For this review, use the dimensioned drawing (mm, ordinates from the lowest corner) and the shaded views. Give positions to 0.01 mm unless a question says otherwise; leave off trailing zeros. Loops run counter-clockwise (first coordinate to the right, second up) from the corner with the lowest first, then second, coordinate; pieces in that order, holes last. Notation, with made-up numbers: M -8,72.5 L 17,72.5 A19 ccw 17,90.5 Z; hole C 50,30 d8. An arc over 180 degrees is marked long. Use a Markdown table: item, result. Add a question column.
(1) Draft analysis for pull direction Y (two halves, no side actions). For the marked faces 1, 2, 3 and 4, state which applies: pulls with the +Y half, pulls with the -Y half, needs draft (parallel to the pull), parting line crosses it, or undercut.
(2) Add section C-C, the plane y = 1.75. Give the boundary of the cut face in (x, z).
(3) For probe 1 along Y at (x, z) = (5, 2.2); probe 2 along X at (y, z) = (6.5, 1.75); probe 3 along Z at (x, y) = (28.5, 0.5), list the stretches that pass through material, from the lowest coordinate up.
(4) Add section B-B, the plane z = 2. Give the boundary of the cut face in (x, y), then the cut area to 3 significant figures.
(5) Add section A-A, the plane x = 5. Give the boundary of the cut face in (y, z), then the cut area to 3 significant figures.
(6) Add section D-D, the plane z = 5.25. Give the boundary of the cut face in (x, y), then the cut area to 3 significant figures.
(7) Insertion check: pin 1 Ø5.5 at (x, y) = (23, 5) entering from -Z; pin 2 Ø2 at (y, z) = (2, 6) entering from -X; pin 3 Ø6 at (x, y) = (14.5, 7.5) entering from +Z. Each pin has a flat end and moves straight along its axis. Give the tip position at first contact, or say it passes through.
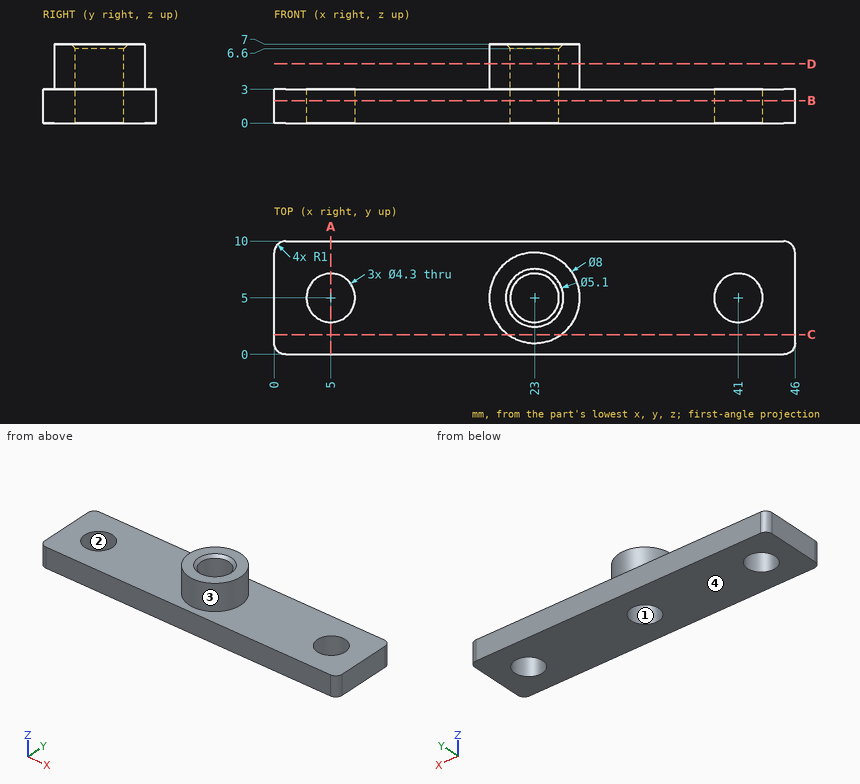
Established:
| question | item | result |
|---|---|---|
| 1 | face 1 | undercut |
| 1 | face 2 | undercut |
| 1 | face 3 | parting line crosses it |
| 1 | face 4 | needs draft |
| 2 | outline | M 0,0 L 46,0 L 46,3 L 25.33,3 L 25.33,7 L 20.67,7 L 20.67,3 L 0,3 Z |
| 3 | probe 1 | 0 to 2.85, 7.15 to 10 |
| 3 | probe 2 | 0 to 3.46, 6.54 to 21.46, 24.54 to 39.46, 42.54 to 46 |
| 3 | probe 3 | 0 to 3 |
| 4 | outline | M 0,1 A1 ccw 1,0 L 45,0 A1 ccw 46,1 L 46,9 A1 ccw 45,10 L 1,10 A1 ccw 0,9 Z; hole C 5,5 d4.3; hole C 23,5 d4.3; hole C 41,5 d4.3 |
| 4 | area | 416 mm^2 |
| 5 | outline | M 0,0 L 2.85,0 L 2.85,3 L 0,3 Z; M 7.15,0 L 10,0 L 10,3 L 7.15,3 Z |
| 5 | area | 17.1 mm^2 |
| 6 | outline | C 23,5 d8; hole C 23,5 d4.3 |
| 6 | area | 35.7 mm^2 |
| 7 | pin 1 | z = 0 |
| 7 | pin 2 | x = 19.54 |
| 7 | pin 3 | z = 3 |
